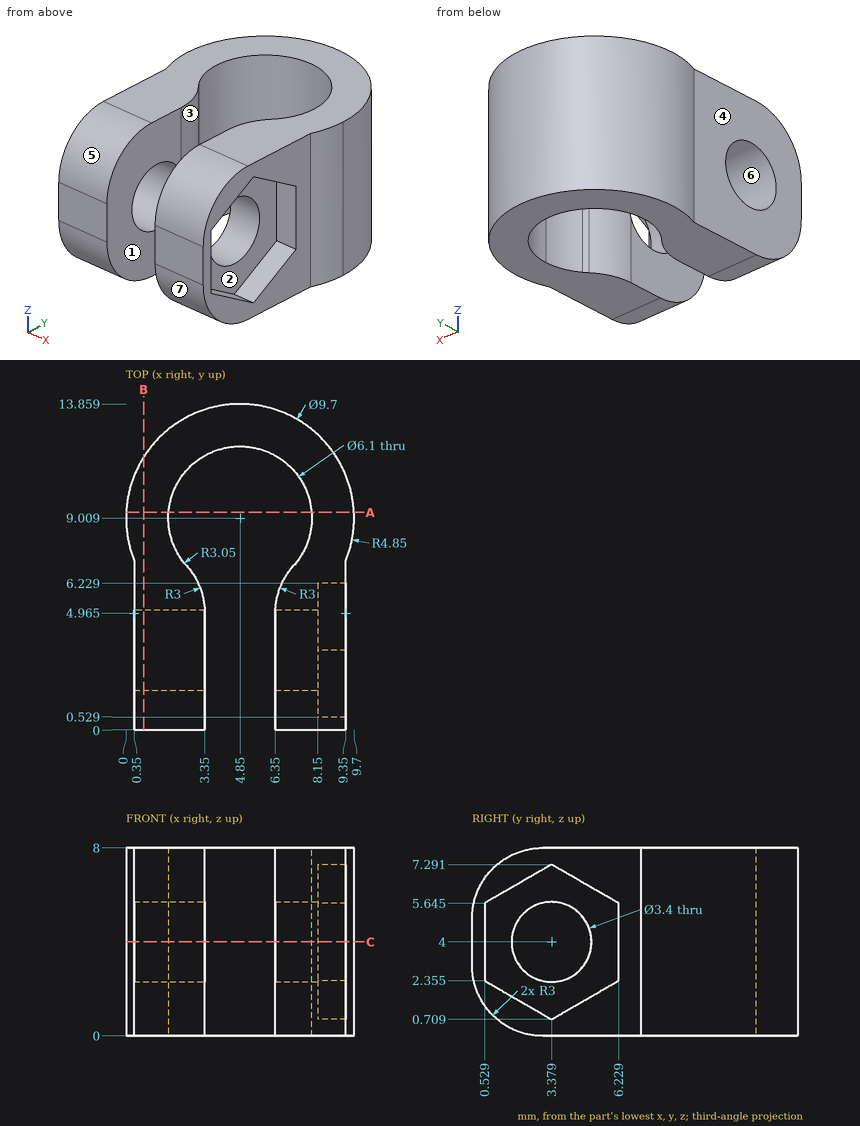
Input: dimensioned drawing with shaded views. Units: mm. Origin: part minimum x, y, z. A direction names the side the tool comes from. Give positions to 0.01 mm unless a question says otherwise; leave off trailing zeros. Order: outer loops, then holes, each group sorted by start corner. A loop starts at its lowest first (then second) coordinate and runs counter-clockwise, first axis right, second up. Notation, with made-up numbers: (-14, 15) -> (43, 15) arc R23 cw to (43, 28) -> close; hole circle Ø7 at (-5.5, 43). An arc over 180 degrees is marked (long way). Use a Markdown table: item, result.
1) Section query A-A, the plane y = 9.25. Return the cut outline in (x, z).
Answer list:
| item | result |
|---|---|
| outline | (0.01, 0) -> (1.81, 0) -> (1.81, 8) -> (0.01, 8) -> close; (7.89, 0) -> (9.69, 0) -> (9.69, 8) -> (7.89, 8) -> close |
2) Ray query, line 1 along X through (y, z) = (2, 5.5); line 2 along Z through (x, y) = (2.75, 3.5) (1 decimal); line 3 along Y through (x, z) = (6.75, 2.5) (1 decimal). Return the intervals inside material, ascending. Write a range as [from, to].
Answer list:
| item | result |
|---|---|
| line 1 | [0.35, 3.35], [6.35, 8.15] |
| line 2 | [0, 2.3], [5.7, 8] |
| line 3 | [0, 2.6], [4.2, 6.5], [11.4, 13.5] |
3) Section query C-C, the plane z = 4. Count the separate pieces of the cut face and the enclosed holes in it.
Answer list:
| item | result |
|---|---|
| separate pieces | 3 |
| enclosed holes | 0 |
4) Reachability of the marked faces 1, 2, 3 and 4 from +Z, -Z, +X, -X, +Y, -Y: full face, straight path, thin tool, end or side. Return the list, or none.
Answer list:
| item | result |
|---|---|
| face 1 | +Z, -Z, -Y |
| face 2 | +X |
| face 3 | +Z, -Z |
| face 4 | +Z, -Z, -X, -Y |
5) Mould query, pull axis Z, two halves, no side actions, for the marked faces 5, 6 and 7. Classes: +Z half, -Z half, draft (parallel to the pull), parting line (faces both ways), or undercut.
Answer list:
| item | result |
|---|---|
| face 5 | +Z half |
| face 6 | undercut |
| face 7 | -Z half |
6) Section query B-B, the plane x = 0.75. Return the cut outline in (y, z).
Answer list:
| item | result |
|---|---|
| outline | (0, 3) arc R3 ccw to (3, 0) -> (11.6, 0) -> (11.6, 8) -> (3, 8) arc R3 ccw to (0, 5) -> close; hole circle Ø3.4 at (3.38, 4) |
7) Contact query for flat-ended pins moving along their axis: P1, Ø2, axis at x = 6.5, z = 1, coming from the -Y side; P2, Ø2, axis at x = 3.5, z = 2.5, coming from the +Y side; P3, Ø3, axis at x = 7.5, z = 7, coming from the -Y side. Output: stop coordinate, or through.
Answer list:
| item | result |
|---|---|
| P1 | y = 0.17 |
| P2 | y = 13.85 |
| P3 | y = 0.04 |
